The listing builds one solid part. Answer for the finished solid, in the listing's coordinates (mm). A direction names the side the tool comes from. Coordinates: 2 decimals unless noted, no trailing zeros. Write each loop counter-clockwise with the first axis right and the second up, starting at its lowest first coordinate (ties: lowest second). Pieces come first, ordered by that corner, then holes.
(1) Given P1, Ø2, axis at y = -8.5, z = -3, coming from the +X side; P2, Ø1, axis at x = 3, y = 4.5, coming from the +Z side; P3, Ø3, axis at y = 6, z = 9, coming from the -X side, each flat-ended and moving along its own axis, determine where each tip first touches the part or whether it passes through.
(2) Straight lines are drawn through the part: line 1 (X direction, y = 10.75, z = -0.75); line 2 (Z direction, x = -13, y = 0.25); line 3 (X direction, y = -10.25, z = 9.5). For each, find the intervals that lie inside material, in ascending order.
(3) The part is cut by section A-A on y = -9.5. Determine the outline of the cut face in (x, z), plus the area to 3 significant figures.
(4) Which of the six approach directions +Z, -Z, +X, -X, +Y, -Y give full straight-line access (tool end or side, diameter ignored) to faces 5 (the cylindrical face through (-20, 12.2, 0.2)), 6 (the flat face through (-17, 12.5, 0)), 7 (the cylindrical face through (-20, -12.2, 0.2)), 8 (the flat face through (21, -12, 0))?
(5) The part is cut by section B-B on z = -8.5. Determine the outline of the cut face in (x, y), plus the area to 3 significant figures.
(6) The part is cut by section D-D on z = 3.75. Determine the outline of the cut face in (x, y).
(7) The part is cut by section C-C on y = 0. Determine the outline of the cut face in (x, z).
(8) For a pull along X with two mould halves and no side action, classify faces 1 (the flat face through (15, -6, 6)), 2 (the flat face through (21, 12, 0)), 3 (the flat face through (-15, -6, 6)), 4 (the cylindrical face through (-24.5, 0.2, 0.2)) as +X half, -X half, draft (parallel to the pull), parting line (faces both ways), or undercut.
from build123d import *

# Parameters (mm, degrees)
F1_START      = -15
F0_W          = 25
F0_H          = 25
F0_R          = 7.5
F1_DEPTH      = 10
F2_START      = 15
F2_DEPTH      = 10
F3_DEPTH      = 16
F3_DEPTH_BACK = 16
F5_START      = -25
F4_R          = 24.5
F5_DEPTH      = 50
F7_START      = -12
F6_R          = 37.8818681869
F6_R_2        = 20
F7_DEPTH      = 13
F8_START      = 12
F8_DEPTH      = 13


with BuildPart() as f1:
    # F0 (on Right) → F1 (new body)
    with BuildSketch(Plane.YZ.offset(F1_START)):
        Rectangle(F0_W, F0_H)
        Circle(F0_R, mode=Mode.SUBTRACT)
        Circle(F0_R)
    extrude(amount=-F1_DEPTH)



with BuildPart() as f2:
    # F0 (on Right) → F2 (new body)
    with BuildSketch(Plane.YZ.offset(F2_START)):
        Rectangle(F0_W, F0_H)
        Circle(F0_R, mode=Mode.SUBTRACT)
        Circle(F0_R)
    extrude(amount=F2_DEPTH)


with BuildPart() as f1_1:
    add(f1.part)

    add(f2.part)  # F3 merges F2
    # F0 (on Right) → F3 (join, two sides)
    with BuildSketch(Plane.YZ) as f3_sk:
        Circle(F0_R)
    extrude(amount=F3_DEPTH)
    extrude(f3_sk.sketch, amount=-F3_DEPTH_BACK)

    # F4 (on Front) → F5 (intersect)
    with BuildSketch(Plane.XZ.offset(F5_START)):
        Circle(F4_R)
    extrude(amount=F5_DEPTH, mode=Mode.INTERSECT)

    # F6 (on Front) → F7 (cut)
    with BuildSketch(Plane.XZ.offset(F7_START)):
        Circle(F6_R)
        Circle(F6_R_2, mode=Mode.SUBTRACT)
    extrude(amount=-F7_DEPTH, mode=Mode.SUBTRACT)

    # F6 (on Front) → F8 (cut)
    with BuildSketch(Plane.XZ.offset(F8_START)):
        Circle(F6_R)
        Circle(F6_R_2, mode=Mode.SUBTRACT)
    extrude(amount=F8_DEPTH, mode=Mode.SUBTRACT)


solid = f1_1.part
Model answer:
1. P1: stops at x = 24.42
1. P2: stops at z = 6.34
1. P3: stops at x = -23.32
2. line 1: x = -24.49 to -15, 15 to 24.49
2. line 2: z = -7.5 to 7.5
2. line 3: x = -22.58 to -15, 15 to 22.58
3. outline: (-21.07, -12.5) - (-15, -12.5) - (-15, 12.5) - (-21.07, 12.5) arc R24.5 ccw to start; (15, -12.5) - (21.07, -12.5) arc R24.5 ccw to (21.07, 12.5) - (15, 12.5) - close
3. area: 420 mm2
4. face 5: -X, +Y
4. face 6: +Z, -Z, +X, -X, +Y
4. face 7: -X, -Y
4. face 8: +X, -Y
5. outline: (-22.98, -12) - (-18.1, -12) - (-18.1, -12.5) - (-15, -12.5) - (-15, 12.5) - (-18.1, 12.5) - (-18.1, 12) - (-22.98, 12) - close; (15, -12.5) - (18.1, -12.5) - (18.1, -12) - (22.98, -12) - (22.98, 12) - (18.1, 12) - (18.1, 12.5) - (15, 12.5) - close
5. area: 389 mm2
6. outline: (-24.21, -12) - (-19.65, -12) - (-19.65, -12.5) - (-15, -12.5) - (-15, -6.5) - (15, -6.5) - (15, -12.5) - (19.65, -12.5) - (19.65, -12) - (24.21, -12) - (24.21, 12) - (19.65, 12) - (19.65, 12.5) - (15, 12.5) - (15, 6.5) - (-15, 6.5) - (-15, 12.5) - (-19.65, 12.5) - (-19.65, 12) - (-24.21, 12) - close
7. outline: (-21.07, -12.5) - (-15, -12.5) - (-15, -7.5) - (15, -7.5) - (15, -12.5) - (21.07, -12.5) arc R24.5 ccw to (21.07, 12.5) - (15, 12.5) - (15, 7.5) - (-15, 7.5) - (-15, 12.5) - (-21.07, 12.5) arc R24.5 ccw to start
8. face 1: undercut
8. face 2: draft
8. face 3: undercut
8. face 4: -X half
